```python
from build123d import *

# Parameters (mm, degrees)
F0_R         = 3
F0_R_2       = 1.5
F1_DEPTH     = 2.4
F2_DEPTH     = 1
F3_T1_DEPTH  = 1.1190522621
F3_T3_DEPTH  = 32.4
F3_T5_DEPTH  = 20.138628613
F3_T7_DEPTH  = 2.365520331
F3_T9_DEPTH  = 8.3614446785
F3_T11_DEPTH = 8.3614446785
F3_T13_DEPTH = 5.1
F3_T15_DEPTH = 2.5639483811
F3_T20_DEPTH = 1.8
F3_S25_W     = 1.8
F3_S25_H     = 1.8
F3_T26_DEPTH = 1.8
F3_S31_W     = 1.8
F3_S31_H     = 1.8
F3_T32_DEPTH = 1.8
F3_T38_DEPTH = 1.8
F3_T44_DEPTH = 1.8
F3_T50_DEPTH = 1.8


# Not quite as in the source:
# - a fillet or chamfer that OpenCascade refuses, or shapes differently, is made with other operations: its cross-section is extruded or revolved along the edge and cut away or added


with BuildPart() as f1:
    # F0 (on Top) → F1 (new body)
    with BuildSketch(Plane.XY):
        Polygon((-18, -1.2002319389), (-18, -4.9048635534), (18, -4.9048635534), (18, -1.2002319389), (10.7755224389, 5.5), (-10.7755224389, 5.5), align=None)
        with Locations((-12, 0)):
            Circle(F0_R, mode=Mode.SUBTRACT)
        with BuildLine():
            ThreePointArc((-2.75, -4), (-6.75, 0), (-2.75, 4))
            Line((-2.75, 4), (2.75, 4))
            ThreePointArc((2.75, 4), (6.75, 0), (2.75, -4))
            Line((2.75, -4), (-2.75, -4))
        make_face(mode=Mode.SUBTRACT)
        with Locations((12, 0)):
            Circle(F0_R, mode=Mode.SUBTRACT)
        with Locations((-12, 0)):
            Circle(F0_R)
        with Locations((-12, 0)):
            Circle(F0_R_2, mode=Mode.SUBTRACT)
        with Locations((12, 0)):
            Circle(F0_R)
        with Locations((12, 0)):
            Circle(F0_R_2, mode=Mode.SUBTRACT)
    extrude(amount=F1_DEPTH)

    # F0 (on Top) → F2 (cut)
    with BuildSketch(Plane.XY):
        with Locations((12, 0)):
            Circle(F0_R)
        with Locations((12, 0)):
            Circle(F0_R_2, mode=Mode.SUBTRACT)
        with Locations((-12, 0)):
            Circle(F0_R)
        with Locations((-12, 0)):
            Circle(F0_R_2, mode=Mode.SUBTRACT)
    extrude(amount=F2_DEPTH, mode=Mode.SUBTRACT)

    # F3: fillet of radius 1.8 on 12 edges, made by hand

    # F3_s2 → F3_t1 (cut)
    with BuildSketch(Plane.XZ.offset(1.9858112913)):
        with BuildLine():
            ThreePointArc((-18, 1.8), (-17.4727922061, 0.5272077939), (-16.2, 0))
            Line((-16.2, 0), (-18, 0))
            Line((-18, 0), (-18, 1.8))
        make_face()
        with BuildLine():
            ThreePointArc((16.2, 0), (17.4727922061, 0.5272077939), (18, 1.8))
            Line((18, 1.8), (18, 0))
            Line((18, 0), (16.2, 0))
        make_face()
    extrude(amount=F3_T1_DEPTH, mode=Mode.SUBTRACT)

    # F3_s4 → F3_t3 (cut)
    with BuildSketch(Plane.YZ.offset(-16.2)):
        with BuildLine():
            ThreePointArc((-4.9048635534, 1.8), (-4.3776557595, 0.5272077939), (-3.1048635534, 0))
            Line((-3.1048635534, 0), (-4.9048635534, 0))
            Line((-4.9048635534, 0), (-4.9048635534, 1.8))
        make_face()
    extrude(amount=F3_T3_DEPTH, mode=Mode.SUBTRACT)

    # F3_s6 → F3_t5 (cut)
    with BuildSketch(Plane.YZ.offset(-10.0693143065)):
        with BuildLine():
            ThreePointArc((3.7, 0), (4.9727922061, 0.5272077939), (5.5, 1.8))
            Line((5.5, 1.8), (5.5, 0))
            Line((5.5, 0), (3.7, 0))
        make_face()
    extrude(amount=F3_T5_DEPTH, mode=Mode.SUBTRACT)

    # F3_s8 → F3_t7 (cut)
    with BuildSketch(Plane.XY.offset(1.8)):
        with BuildLine():
            ThreePointArc((10.0693143065, 5.5), (10.7267347006, 5.3756486581), (11.2933205301, 5.0197760282))
            Line((11.2933205301, 5.0197760282), (10.7755224389, 5.5))
            Line((10.7755224389, 5.5), (10.0693143065, 5.5))
        make_face()
        with BuildLine():
            ThreePointArc((-11.2933205301, 5.0197760282), (-10.7267347006, 5.3756486581), (-10.0693143065, 5.5))
            Line((-10.0693143065, 5.5), (-10.7755224389, 5.5))
            Line((-10.7755224389, 5.5), (-11.2933205301, 5.0197760282))
        make_face()
    extrude(amount=F3_T7_DEPTH, mode=Mode.SUBTRACT)

    # F3_s10 → F3_t9 (cut)
    with BuildSketch(Plane(origin=(-3.5684530391, -3.3095075488, 0), x_dir=(0, 0, 1), z_dir=(-0.7332089046, -0.6800034575, 0))):
        with BuildLine():
            ThreePointArc((1.8, 11.3600414903), (0.5272077939, 10.8328336964), (0, 9.5600414903))
            Line((0, 9.5600414903), (0, 11.3600414903))
            Line((0, 11.3600414903), (1.8, 11.3600414903))
        make_face()
    extrude(amount=F3_T9_DEPTH, mode=Mode.SUBTRACT)

    # F3_s12 → F3_t11 (cut)
    with BuildSketch(Plane(origin=(9.6991387326, -8.9953188401, 0), x_dir=(0, 0, 1), z_dir=(-0.7332089046, 0.6800034575, 0))):
        with BuildLine():
            ThreePointArc((0, 9.5600414903), (0.5272077939, 10.8328336964), (1.8, 11.3600414903))
            Line((1.8, 11.3600414903), (0, 11.3600414903))
            Line((0, 11.3600414903), (0, 9.5600414903))
        make_face()
    extrude(amount=F3_T11_DEPTH, mode=Mode.SUBTRACT)

    # F3_s14 → F3_t13 (cut)
    with BuildSketch(Plane.XY.offset(1.8)):
        with BuildLine():
            ThreePointArc((-18, -3.1048635534), (-17.4727922061, -4.3776557595), (-16.2, -4.9048635534))
            Line((-16.2, -4.9048635534), (-18, -4.9048635534))
            Line((-18, -4.9048635534), (-18, -3.1048635534))
        make_face()
        with BuildLine():
            ThreePointArc((16.2, -4.9048635534), (17.4727922061, -4.3776557595), (18, -3.1048635534))
            Line((18, -3.1048635534), (18, -4.9048635534))
            Line((18, -4.9048635534), (16.2, -4.9048635534))
        make_face()
    extrude(amount=F3_T13_DEPTH, mode=Mode.SUBTRACT)

    # F3_s16 → F3_t15 (cut)
    with BuildSketch(Plane.XY.offset(1.8)):
        with BuildLine():
            ThreePointArc((-18, -1.9858112913), (-17.8497289478, -1.265815181), (-17.4240062235, -0.666035263))
            Line((-17.4240062235, -0.666035263), (-18, -1.2002319389))
            Line((-18, -1.2002319389), (-18, -1.9858112913))
        make_face()
        with BuildLine():
            ThreePointArc((18, -1.9858112913), (17.8497289478, -1.265815181), (17.4240062235, -0.666035263))
            Line((17.4240062235, -0.666035263), (18, -1.2002319389))
            Line((18, -1.2002319389), (18, -1.9858112913))
        make_face()
    extrude(amount=F3_T15_DEPTH, mode=Mode.SUBTRACT)


with BuildPart() as f3_tool18:
    # F3_s19 → F3_t20 (new body)
    with BuildSketch(Plane.XY.offset(1.8)):
        Polygon((-16.2, -1.9858112913), (-18, -1.9858112913), (-18, -1.2002319389), (-17.4240062235, -0.666035263), align=None)
    extrude(amount=-F3_T20_DEPTH)

    # F3_s21 → F3_t22 (revolve, cut)
    with BuildSketch(Plane(origin=(-16.2, -1.9858112913, 1.8), x_dir=(0.9165160821, -0.399997839, 0), z_dir=(0.399997839, 0.9165160821, 0))):
        with BuildLine():
            ThreePointArc((0, -1.8), (1.8, 0), (0, 1.8))
            Line((0, 1.8), (0, -1.8))
        make_face()
    revolve(axis=Axis((-16.2, -1.9858112913, 1.8), (0, 0, -1)), mode=Mode.SUBTRACT)


with BuildPart() as f1_1:
    add(f1.part)

    # F3_t17: cut F3_tool18
    add(f3_tool18.part, mode=Mode.SUBTRACT)


with BuildPart() as f3_tool24:
    # F3_s25 → F3_t26 (new body)
    with BuildSketch(Plane.YZ.offset(-16.2)):
        with Locations((-4.0048635534, 0.9)):
            Rectangle(F3_S25_W, F3_S25_H)
    extrude(amount=-F3_T26_DEPTH)

    # F3_s27 → F3_t28 (revolve, cut)
    with BuildSketch(Plane(origin=(-16.2, -3.1048635534, 1.8), x_dir=(0, 0.7071067812, 0.7071067812), z_dir=(0, -0.7071067812, 0.7071067812))):
        with BuildLine():
            ThreePointArc((0, -1.8), (1.8, 0), (0, 1.8))
            Line((0, 1.8), (0, -1.8))
        make_face()
    revolve(axis=Axis((-16.2, -3.1048635534, 1.8), (-1, 0, 0)), mode=Mode.SUBTRACT)


with BuildPart() as f1_2:
    add(f1_1.part)

    # F3_t23: cut F3_tool24
    add(f3_tool24.part, mode=Mode.SUBTRACT)


with BuildPart() as f3_tool30:
    # F3_s31 → F3_t32 (new body)
    with BuildSketch(Plane.XZ.offset(3.1048635534)):
        with Locations((17.1, 0.9)):
            Rectangle(F3_S31_W, F3_S31_H)
    extrude(amount=F3_T32_DEPTH)

    # F3_s33 → F3_t34 (revolve, cut)
    with BuildSketch(Plane(origin=(16.2, -3.1048635534, 1.8), x_dir=(-0.7071067812, 0, 0.7071067812), z_dir=(0.7071067812, 0, 0.7071067812))):
        with BuildLine():
            ThreePointArc((0, -1.8), (1.8, 0), (0, 1.8))
            Line((0, 1.8), (0, -1.8))
        make_face()
    revolve(axis=Axis((16.2, -3.1048635534, 1.8), (0, -1, 0)), mode=Mode.SUBTRACT)


with BuildPart() as f1_3:
    add(f1_2.part)

    # F3_t29: cut F3_tool30
    add(f3_tool30.part, mode=Mode.SUBTRACT)


with BuildPart() as f3_tool36:
    # F3_s37 → F3_t38 (new body)
    with BuildSketch(Plane.XY.offset(1.8)):
        Polygon((16.2, -1.9858112913), (18, -1.9858112913), (18, -1.2002319389), (17.4240062235, -0.666035263), align=None)
    extrude(amount=-F3_T38_DEPTH)

    # F3_s39 → F3_t40 (revolve, cut)
    with BuildSketch(Plane(origin=(16.2, -1.9858112913, 1.8), x_dir=(-0.9165160821, -0.399997839, 0), z_dir=(0.399997839, -0.9165160821, 0))):
        with BuildLine():
            ThreePointArc((0, -1.8), (1.8, 0), (0, 1.8))
            Line((0, 1.8), (0, -1.8))
        make_face()
    revolve(axis=Axis((16.2, -1.9858112913, 1.8), (0, 0, -1)), mode=Mode.SUBTRACT)


with BuildPart() as f1_4:
    add(f1_3.part)

    # F3_t35: cut F3_tool36
    add(f3_tool36.part, mode=Mode.SUBTRACT)


with BuildPart() as f3_tool42:
    # F3_s43 → F3_t44 (new body)
    with BuildSketch(Plane.XY.offset(1.8)):
        Polygon((10.0693143065, 3.7), (10.0693143065, 5.5), (10.7755224389, 5.5), (11.2933205301, 5.0197760282), align=None)
    extrude(amount=-F3_T44_DEPTH)

    # F3_s45 → F3_t46 (revolve, cut)
    with BuildSketch(Plane(origin=(10.0693143065, 3.7, 1.8), x_dir=(-0.3652335523, -0.9309159212, 0), z_dir=(0.9309159212, -0.3652335523, 0))):
        with BuildLine():
            ThreePointArc((0, -1.8), (1.8, 0), (0, 1.8))
            Line((0, 1.8), (0, -1.8))
        make_face()
    revolve(axis=Axis((10.0693143065, 3.7, 1.8), (0, 0, -1)), mode=Mode.SUBTRACT)


with BuildPart() as f1_5:
    add(f1_4.part)

    # F3_t41: cut F3_tool42
    add(f3_tool42.part, mode=Mode.SUBTRACT)


with BuildPart() as f3_tool48:
    # F3_s49 → F3_t50 (new body)
    with BuildSketch(Plane.XY.offset(1.8)):
        Polygon((-10.0693143065, 3.7), (-10.0693143065, 5.5), (-10.7755224389, 5.5), (-11.2933205301, 5.0197760282), align=None)
    extrude(amount=-F3_T50_DEPTH)

    # F3_s51 → F3_t52 (revolve, cut)
    with BuildSketch(Plane(origin=(-10.0693143065, 3.7, 1.8), x_dir=(0.3652335523, -0.9309159212, 0), z_dir=(0.9309159212, 0.3652335523, 0))):
        with BuildLine():
            ThreePointArc((0, -1.8), (1.8, 0), (0, 1.8))
            Line((0, 1.8), (0, -1.8))
        make_face()
    revolve(axis=Axis((-10.0693143065, 3.7, 1.8), (0, 0, -1)), mode=Mode.SUBTRACT)


with BuildPart() as f1_6:
    add(f1_5.part)

    # F3_t47: cut F3_tool48
    add(f3_tool48.part, mode=Mode.SUBTRACT)


solid = f1_6.part
```
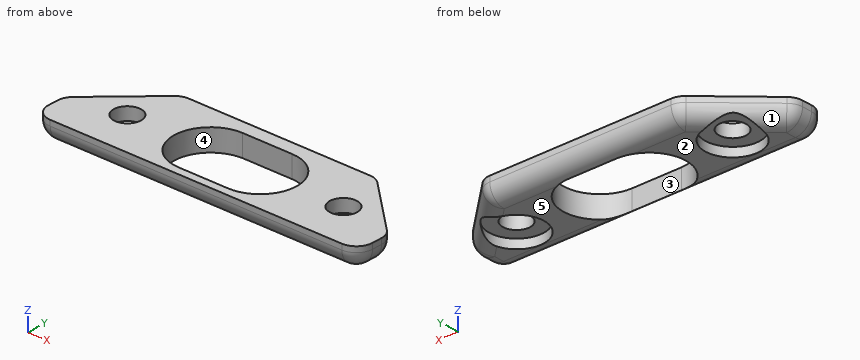
Here's how the part is built. I have some questions about the finished solid (model axes, mm). Face numbers are marked on the shaded views. A direction names the side the tool comes from. Give positions to 0.01 mm unless a question says otherwise; leave off trailing zeros. Loops run counter-clockwise (first coordinate to the right, second up) from the corner with the lowest first, then second, coordinate; pieces in that order, holes last. Notation, with made-up numbers: M 78.5,75 L 108.5,75 A23 cw 108.5,88 Z; hole C 2.5,10 d7. An arc over 180 degrees is marked long. Put each result on its own line as item: value. Start each with the question number.
(1) For the marked faces 4 and 5, which set-ups out of +Z, -Z, +X, -X, +Y, -Y let a thin tool reach every point of the face, with its end or its side?
(2) If we mould it in two halves opening along X, with no side actions, what happens to the marked faces 1, 2 and 3? For each: +X half, -X half, draft (parallel to the pull), parting line (faces both ways), or undercut.
(3) I want a section at B-B on y = 1. State how many separate pieces and enclosed holes the cut face has, then the cut area to 3 significant figures.
(4) Will these pins go through, and if not, where does the flat tip stop? pin 1 Ø3 at (x, y) = (13, -1) entering from -Z; pin 2 Ø1.2 at (x, z) = (0.5, 1) entering from -Y; pin 3 Ø1 at (x, z) = (-12, 2) entering from +Y.
(5) I need wall thicknesses on line 1 along X through (y, z) = (0, 0.4); line 2 along Z through (x, y) = (4.5, 4); line 3 along Z through (x, y) = (-13, 1.75). Which ranges of each line are inside material? Lowest first, please. Write a range as [from, to].
(6) I want a section at A-A on x = -0.5. Please give me the cut outline in (y, z).
Answer block:
1. face 4: +Z, -Z
1. face 5: -Z, +X, -X, +Y, -Y
2. face 1: -X half
2. face 2: draft
2. face 3: undercut
3. separate pieces: 4
3. enclosed holes: 0
3. area: 24.2 mm^2
4. pin 1: z = 1
4. pin 2: y = -4.89
4. pin 3: y = 4.83
5. line 1: [-15.72, -15], [-9, -6.75], [6.75, 9], [15, 15.72]
5. line 2: [0.03, 2.4]
5. line 3: [1, 2.4]
6. outline: M -4.9,1.8 A1.8 ccw -4,0.24 L -4,2.4 L -4.9,2.4 Z; M 4,0.03 A1.8 ccw 5.5,1.8 L 5.5,2.4 L 4,2.4 Z
